Autodesk Inventor part; units mm, degrees
ref_plane "YZ Plane" through (0, 0, 0) normal (1, 0, 0) x (0, 1, 0)
ref_plane "XZ Plane" through (0, 0, 0) normal (0, 1, 0) x (-1, 0, 0)
ref_plane "XY Plane" through (0, 0, 0) normal (0, 0, 1) x (1, 0, 0)
sketch "スケッチ1" plane through (0, 0, 0) normal (0, 0, 1) x (1, 0, 0)
  line L0 (50, -5) -> (-110.2322, -5)
  line L1 (-110.2322, -5) -> (-110.2322, 70.4763)
  line L2 (-110.2322, 70.4763) -> (50, 70.4763)
  line L3 (50, 70.4763) -> (50, -5)
  circle A0 centre (44, 0) radius 2.75
  circle A1 centre (6, 0) radius 2.75
  point P0 (0, 0)
extrude "押し出し1" add sketch "スケッチ1" along normal blind 10
For this review, take the finished solid that the model builds, in its own axes (mm). Round coordinates to 2 decimals unless told otherwise and drop trailing zeros. Write each loop counter-clockwise with the first axis right and the second up, starting at its lowest first coordinate (ties: lowest second). Pieces come first, ordered by that corner, then holes. Notation, with made-up numbers: (24.5, -6.75) -> (52.5, -6.75) arc R18 cw to (52.5, 21.25) -> close; hole circle Ø8 at (63.25, 68.25). An arc over 180 degrees is marked (long way). Use one line per item in the form item = value.
Q1. The part is to be moulded in two halves that separate along X. For faces 1 (the flat face through (-31, 33, 10)), 2 (the cylindrical face through (8.54, 1.05, 4.93)), 3 (the flat face through (50, 33, 5)), say which applies: released by +X, released by -X, zero draft, split by the parting line, or undercut.
Resolved:
face_1 = zero draft
face_2 = undercut
face_3 = released by +X
Q2. To check wall thickness, follow probe 1 along Y at (x, z) = (44, 6); probe 2 along X at (y, z) = (-0.5, 8.5). State the ranges of each line that lie inside material, in increasing order. Write a range as from..to.
Resolved:
probe_1 = -5..-2.75, 2.75..70.48
probe_2 = -110.23..3.3, 8.7..41.3, 46.7..50
Q3. Consider section A-A (y = 0). State the section outline as (x, z) points.
Resolved:
outline = (-110.23, 0) -> (3.25, 0) -> (3.25, 10) -> (-110.23, 10) -> close; (8.75, 0) -> (41.25, 0) -> (41.25, 10) -> (8.75, 10) -> close; (46.75, 0) -> (50, 0) -> (50, 10) -> (46.75, 10) -> close
Q4. Consider section B-B (x = 6). State the section outline as (y, z) points, then the cut area to 3 significant figures.
Resolved:
outline = (-5, 0) -> (-2.75, 0) -> (-2.75, 10) -> (-5, 10) -> close; (2.75, 0) -> (70.48, 0) -> (70.48, 10) -> (2.75, 10) -> close
area = 700 mm²
